The model under review builds one solid part; all positions refer to its coordinate system, in mm. Round coordinates to 2 decimals unless told otherwise and drop trailing zeros. Order: outer loops, then holes, each group sorted by start corner. A loop starts at its lowest first (then second) coordinate and runs counter-clockwise, first axis right, second up. Notation, with made-up numbers: M 63,57.5 L 119,57.5 A27 cw 119,87.5 Z; hole C 42.5,-19.5 d4. An arc over 180 degrees is marked long. Answer as a JSON object with one key per item and string values. Group by question number.
1) Insertion check: pin 1 Ø1 at (y, z) = (-14, 2) entering from -X; pin 2 Ø1 at (y, z) = (-35.5, 2) entering from +X. Each pin has a flat end and moves straight along its axis. Give the tip position at first contact, or say it passes through.
2) To check wall thickness, follow line 1 (Y direction, x = -17.5, z = 1.5); line 2 (X direction, y = -13.5, z = 1.15); line 3 (X direction, y = -1.5, z = 0.95). State the ranges of each line that lie inside material, in increasing order.
3) Consider section C-C, the plane x = -37. Write out the cut boundary in (y, z) (3 decimals), then the cut area to 3 significant figures.
4) Consider section D-D, the plane y = -20. Write out the cut boundary in (x, z) (3 decimals), then the cut area to 3 significant figures.
5) Consider section A-A, the plane y = -28.25. Write out the cut boundary in (x, z) (3 decimals).
6) Consider section B-B, the plane x = -17.5. Write out the cut boundary in (y, z) (3 decimals).
```python
from build123d import *

# Parameters (mm, degrees)
SKETCH1_R           = 32
SKETCH1_R_2         = 25
SKETCH1_R_3         = 1.4732
BOSS_EXTRUDE1_DEPTH = 3.175


with BuildPart() as part:
    # Sketch1 → Boss-Extrude1 (new body)
    with BuildSketch(Plane.XY.offset(0.2)):
        with Locations((-17.5, -28.25)):
            Circle(SKETCH1_R)
        with Locations((-17.5, -28.25)):
            Circle(SKETCH1_R_2, mode=Mode.SUBTRACT)
        with Locations((-17.5, -55.7)):
            Circle(SKETCH1_R_3, mode=Mode.SUBTRACT)
        with Locations((-31.225, -52.022397334)):
            Circle(SKETCH1_R_3, mode=Mode.SUBTRACT)
        with Locations((-41.272397334, -41.975)):
            Circle(SKETCH1_R_3, mode=Mode.SUBTRACT)
        with Locations((-44.95, -28.25)):
            Circle(SKETCH1_R_3, mode=Mode.SUBTRACT)
        with Locations((-41.272397334, -14.525)):
            Circle(SKETCH1_R_3, mode=Mode.SUBTRACT)
        with Locations((-31.225, -4.477602666)):
            Circle(SKETCH1_R_3, mode=Mode.SUBTRACT)
        with Locations((-17.5, -0.8)):
            Circle(SKETCH1_R_3, mode=Mode.SUBTRACT)
        with Locations((-3.775, -4.477602666)):
            Circle(SKETCH1_R_3, mode=Mode.SUBTRACT)
        with Locations((6.272397334, -14.525)):
            Circle(SKETCH1_R_3, mode=Mode.SUBTRACT)
        with Locations((9.95, -28.25)):
            Circle(SKETCH1_R_3, mode=Mode.SUBTRACT)
        with Locations((6.272397334, -41.975)):
            Circle(SKETCH1_R_3, mode=Mode.SUBTRACT)
        with Locations((-3.775, -52.022397334)):
            Circle(SKETCH1_R_3, mode=Mode.SUBTRACT)
    extrude(amount=BOSS_EXTRUDE1_DEPTH)


solid = part.part
```
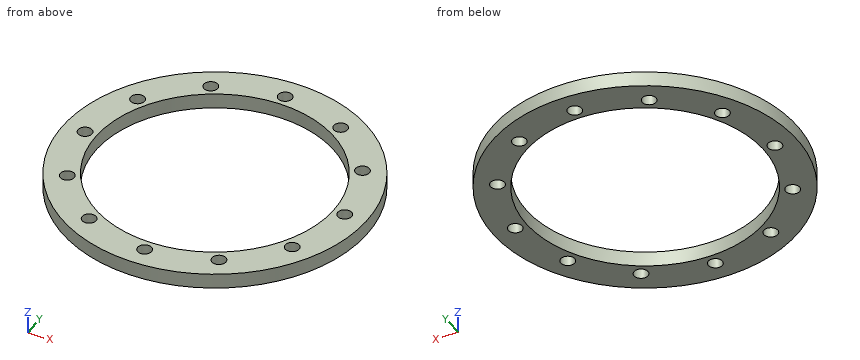
Results list:
{
 "1": {"pin 1": "x = -46.4", "pin 2": "x = 13.78"},
 "2": {"line 1": "-60.25 to -57.17, -54.23 to -53.25, -3.25 to -2.27, 0.67 to 3.75", "line 2": "-45.9 to -42.33, -40.21 to -37.69, 2.69 to 5.21, 7.33 to 10.9", "line 3": "-35.06 to -18.8, -16.2 to 0.06"},
 "3": {"outline": "M -53.622,0.2 L -43.894,0.2 L -43.894,3.375 L -53.622,3.375 Z; M -12.606,0.2 L -2.878,0.2 L -2.878,3.375 L -12.606,3.375 Z", "area": "61.8 mm^2"},
 "4": {"outline": "M -48.418,0.2 L -41.1,0.2 L -41.1,3.375 L -48.418,3.375 Z; M 6.1,0.2 L 13.418,0.2 L 13.418,3.375 L 6.1,3.375 Z", "area": "46.5 mm^2"},
 "5": {"outline": "M -49.5,0.2 L -46.423,0.2 L -46.423,3.375 L -49.5,3.375 Z; M -43.477,0.2 L -42.5,0.2 L -42.5,3.375 L -43.477,3.375 Z; M 7.5,0.2 L 8.477,0.2 L 8.477,3.375 L 7.5,3.375 Z; M 11.423,0.2 L 14.5,0.2 L 14.5,3.375 L 11.423,3.375 Z"},
 "6": {"outline": "M -60.25,0.2 L -57.173,0.2 L -57.173,3.375 L -60.25,3.375 Z; M -54.227,0.2 L -53.25,0.2 L -53.25,3.375 L -54.227,3.375 Z; M -3.25,0.2 L -2.273,0.2 L -2.273,3.375 L -3.25,3.375 Z; M 0.673,0.2 L 3.75,0.2 L 3.75,3.375 L 0.673,3.375 Z"}
}
